from build123d import *

# Parameters (mm, degrees)
ESQUISSE1_W             = 6
ESQUISSE1_H             = 18
BOSS_EXTRU_1_DEPTH      = 28
ESQUISSE2_R             = 1.6
ENL_V_MAT_EXTRU_1_DEPTH = 28


with BuildPart() as part:
    # Esquisse1 → Boss.-Extru.1 (new body)
    with BuildSketch(Plane.XY):
        Rectangle(ESQUISSE1_W, ESQUISSE1_H)
    extrude(amount=BOSS_EXTRU_1_DEPTH)

    # Esquisse2 → Enlèv. mat.-Extru.1 (cut)
    with BuildSketch(Plane.ZY.offset(3)):
        with Locations((2.5, -6.4)):
            Circle(ESQUISSE2_R)
        with Locations((25.5, -6.4)):
            Circle(ESQUISSE2_R)
    extrude(amount=-ENL_V_MAT_EXTRU_1_DEPTH, mode=Mode.SUBTRACT)


solid = part.part
Source: CAD feature listing. Evaluate the final solid. Frame: model axes, mm. Round coordinates to 2 decimals unless told otherwise and drop trailing zeros. Loops run counter-clockwise (first coordinate to the right, second up) from the corner with the lowest first, then second, coordinate; pieces in that order, holes last. Notation, with made-up numbers: (-31.5, -14) -> (22.5, -14) arc R21 cw to (22.5, 20) -> close; hole circle Ø7 at (-39.5, 26). An arc over 180 degrees is marked (long way). Answer as a JSON object with one key per item and string values. Group by question number.
Q1. Section query A-A (z = 2.5). Output: boundary loops of the cut face in (x, y).
Q2. Ray query, line 1 (Y direction, x = -1, z = 25.5); line 2 (Z direction, x = 2.5, y = -7.25); line 3 (Y direction, x = 0.85, z = 24.5). Return the intervals inside material, ascending. Write a range as from..to.
Q3. Section query C-C (x = -1.1). Output: boundary loops of the cut face in (y, z).
Q4. Section query B-B (y = -7.5). Output: boundary loops of the cut face in (x, z).
Q5. Section query D-D (z = 25). Output: boundary loops of the cut face in (x, y).
Q6. Mould query, pull axis Y, two halves, no side actions, for faces 1 (the flat face through (3, 0, 14)), 2 (the flat face through (0, -9, 14)), 3 (the cylindrical face through (-0.04, -5.32, 24.32)). Classes: pulls with the +Y half, pulls with the -Y half, needs draft (parallel to the pull), parting line crosses it, or undercut.
Completed:
{
 "1": {"outline": "(-3, -9) -> (3, -9) -> (3, -8) -> (-3, -8) -> close; (-3, -4.8) -> (3, -4.8) -> (3, 9) -> (-3, 9) -> close"},
 "2": {"line 1": "-9..-8, -4.8..9", "line 2": "0..1.14, 3.86..24.14, 26.86..28", "line 3": "-9..-7.65, -5.15..9"},
 "3": {"outline": "(-9, 0) -> (9, 0) -> (9, 28) -> (-9, 28) -> close; hole circle Ø3.2 at (-6.4, 2.5); hole circle Ø3.2 at (-6.4, 25.5)"},
 "4": {"outline": "(-3, 0) -> (3, 0) -> (3, 1.34) -> (-3, 1.34) -> close; (-3, 3.66) -> (3, 3.66) -> (3, 24.34) -> (-3, 24.34) -> close; (-3, 26.66) -> (3, 26.66) -> (3, 28) -> (-3, 28) -> close"},
 "5": {"outline": "(-3, -9) -> (3, -9) -> (3, -7.92) -> (-3, -7.92) -> close; (-3, -4.88) -> (3, -4.88) -> (3, 9) -> (-3, 9) -> close"},
 "6": {"face 1": "needs draft", "face 2": "pulls with the -Y half", "face 3": "undercut"}
}
